Can you work these out from the model? Positions are in its coordinate system, mm. A direction names the side the tool comes from. Give positions to 0.01 mm unless a question says otherwise; leave off trailing zeros. Write each loop counter-clockwise with the first axis right and the second up, starting at its lowest first coordinate (ties: lowest second). Pieces come first, ordered by that corner, then holes.
Autodesk Inventor part; units mm, degrees
ref_plane "YZ Plane" through (0, 0, 0) normal (1, 0, 0) x (0, 1, 0)
ref_plane "XZ Plane" through (0, 0, 0) normal (0, 1, 0) x (-1, 0, 0)
ref_plane "XY Plane" through (0, 0, 0) normal (0, 0, 1) x (1, 0, 0)
sketch "Sketch1" plane through (0, 0, 0) normal (1, 0, 0) x (0, 1, 0)
  line L0 (-39.3892, -105) -> (-110, -20.8494)
  line L1 (-110, -20.8494) -> (-110, 0)
  line L2 (-110, 0) -> (0, 0)
  line L3 (0, 0) -> (0, -105)
  line L4 (0, -105) -> (-39.3892, -105)
  line L5 (-110, -20.8494) -> (-119.38, 0) construction
  line L6 (-119.38, 0) -> (-110, 0) construction
  line L7 (-50.8, -25.4) -> (0, -25.4) construction
  line L8 (0, -25.4) -> (0, 0) construction
  line L9 (0, 0) -> (-50.8, 0) construction
  line L10 (-50.8, 0) -> (-50.8, -25.4) construction
  line L11 (-50.8, -25.4) -> (0, 0) construction
  line L12 (0, -25.4) -> (-50.8, 0) construction
  circle A0 centre (-12.7, -12.7) radius 3
  circle A1 centre (-38.1, -12.7) radius 3
  circle A2 centre (-25.4, -75) radius 14.2875
  circle A3 centre (-25.4, -75) radius 30
  line L13 (-50.8, -90.9637) -> (-50.8, -59.0363)
  line L14 (-50.8, -25.4) -> (0, -25.4)
  line L15 (-66.8394, 0) -> (-50.8, -90.9637)
  line L16 (-50.8, -25.4) -> (-50.8, 0)
  point P0 (-25.4, -12.7)
  point P1 (-25.4, -25.4)
  point P2 (-50.8, -75)
  point P3 (0, -90.9637)
  point P4 (0, -25.4)
  point P5 (-50.8, 0)
  dimension "d0" = 50
  dimension "d1" = 119.38
  dimension "d2" = 50.8
  dimension "d3" = 25.4
  dimension "d4" = 25.4
  dimension "d5" = 12.7
  dimension "d6" = 6
  dimension "d7" = 6
  dimension "d11" = 75
  dimension "d13" = 110
  dimension "d16" = 60
  dimension "d17" = 25.4
  dimension "d18" = 25.4
  dimension "d31" = 28.575
  dimension "d33" = 10
extrude "Plate1" add sketch "Sketch1" along normal blind 1.5875 contours A3 L13 L3 | L15 A3 L13 | L15 L2 L16 L14 L3 A3
fillet "Corner Round2" radius 6 4 edges at (0.7937, 0, -90.9637) (0.7937, -50.8, -90.9637) (0.7937, 0, -25.4) (0.7937, -66.8394, 0)
sketch "Sketch3" plane through (0, -50.8, -26.9875) normal (0, 0, 1) x (1, 0, 0)
  line L0 (0, 44.8) -> (0, 1.5875)
  line L1 (0, 1.5875) -> (20, 1.5875)
  line L2 (20, 1.5875) -> (20, 44.8)
  line L3 (20, 44.8) -> (0, 44.8)
edge flange "Flange1" height 20 angle 90 thickness 1.5875 bend radius 1.5875 thickness toward (0, 0, 1) relief straight relief width 1.5875 relief depth 0.7937 edges at (1.5875, -28.4, -25.4) wall of the first edge with corners at (0, -6, -26.9875) (0, -49.2125, -26.9875) (20, -49.2125, -26.9875) (20, -6, -26.9875)
bend "Bend1"
corner "Corner1"
sketch "Sketch4" plane through (1.5875, 0, 0) normal (1, 0, 0) x (0, 0, -1)
  circle A0 centre (75, -25.4) radius 14.2875
  point P0 (0, 0)
  point P1 (100.4, -25.4)
  point P2 (92.9605, -7.4395)
  point P3 (75, 0)
  point P4 (57.0395, -7.4395)
  point P5 (49.6, -25.4)
  point P6 (57.0395, -43.3605)
  point P7 (75, -50.8)
  point P8 (92.9605, -43.3605)
  dimension "d45" = 25.4
  dimension "d48" = 360
hole "Hole2" at (1.5875, -25.4, -100.4) at (1.5875, -7.4395, -92.9605) at (1.5875, -7.4395, -57.0395) at (1.5875, -25.4, -49.6) at (1.5875, -43.3605, -57.0395) at (1.5875, -43.3605, -92.9605) direction (-1, 0, 0) diameter 5.105 depth 1.5875 tip angle 118
sketch "Sketch5" plane through (20, -49.2125, -26.9875) normal (0, 0, -1) x (-1, 0, 0)
  line L0 (0, 0) -> (16.825, 0)
  line L1 (16.825, 0) -> (16.825, 43.2125)
  point P0 (20, 49.2125)
  point P1 (8.9807, 9.8425)
  point P2 (8.9807, 35.2425)
  point P3 (8.4125, 0)
  point P4 (8.9807, 23.8125)
  dimension "d57" = 25.4
  dimension "d58" = 9.8425
  dimension "d67" = 23.8125
  dimension "d68" = 7.8443
hole "Hole3" at (11.0193, -39.37, -26.9875) at (11.0193, -13.97, -26.9875) at (11.0193, -25.4, -26.9875) direction (0, 0, 1) diameter 5.105 end through all
fillet "Corner Round3" radius 6 2 edges at (20, -49.2125, -26.1938) (20, -6, -26.1937)
sketch "Sketch6" plane through (1.5875, 0, 0) normal (1, 0, 0) x (0, 0, -1)
  line L0 (29.3688, -50.8) -> (0, -50.8)
  line L1 (0, -59.6888) -> (0, -50.8)
  point P0 (0, 0)
  point P1 (12.7, -57.15)
  dimension "d69" = 6.35
  dimension "d70" = 12.7
hole "Hole4" at (1.5875, -57.15, -12.7) direction (-1, 0, 0) diameter 5.105 end through all
equation "\"d7\" = d6"
equation "\"d55\" = Thickness"
equation "\"d76\" = Thickness"
equation "\"d14\" = Thickness"
equation "\"d35\" = BendReliefWidth"
equation "\"d36\" = BendReliefDepth"
equation "\"d37\" = MinimumRemnant"
equation "\"d38\" = TransitionRadius"
equation "\"d41\" = BendRadius"
equation "\"d42\" = CornerReliefSize"
equation "\"d43\" = GapSize"
equation "\"d44\" = JacobiRadiusSize"
equation "\"BendRadius\" = Thickness"
equation "\"BendReliefWidth\" = Thickness"
equation "\"BendReliefDepth\" = 0.5 * Thickness"
equation "\"CornerReliefSize\" = 4 * Thickness"
equation "\"MinimumRemnant\" = 2 * Thickness"
equation "\"TransitionRadius\" = BendRadius"
equation "\"JacobiRadiusSize\" = BendRadius"
equation "\"GapSize\" = Thickness"
properties part number "INSIDE_INTAKE_PLATE_MOTOR_MOUNT" material "Aluminum, 6061-T6"
(1) If I drill on L1, parallel to X at y = -54.5, z = -55.5; L2, parallel to Z at x = 14.25, y = -14; L3, parallel to Y at x = 1.5, z = -74, over which ranges is the centre line in solid material (lowest first)?
Returned:
L1: x = 0 to 1.59
L2: z = -26.99 to -25.4
L3: y = -53.79 to -39.65, -11.15 to 0
(2) If we mould it in two halves opening along Y, with no side actions, what happens to faces 1 (the face through (0.8, -25.3, -105)), 2 (the face through (0.783, -54.658, -12.147)), 3 (the face through (10.91, -16.52, -26.18)), 4 (the face through (0.78, -58.41, -47.81))? For each: +Y half, -Y half, draft (parallel to the pull), parting line (faces both ways), or undercut.
Returned:
face 1: parting line
face 2: undercut
face 3: undercut
face 4: -Y half
(3) For faces 5 (the face through (18.289, -7.804, -26.183)), 6 (the face through (7, -6, -26)), 7 (the face through (0.95, -27.91, -26.31)), which set-ups out of +Z, -Z, +X, -X, +Y, -Y let a thin tool reach every point of the face, with its end or its side?
Returned:
face 5: +Z, -Z, +X, +Y
face 6: +Z, +X, -X
face 7: +Z, -X
(4) Imagine slicing it at B-B, the plane z = -12.7. Write out the boundary of the cut face in (x, y).
Returned:
outline: (0, -64.6) - (1.59, -64.6) - (1.59, -59.7) - (0, -59.7) - close; (0, -54.6) - (1.59, -54.6) - (1.59, -50.8) - (0, -50.8) - close
(5) Imagine slicing it at C-C, the plane y = -57.15. Write out the boundary of the cut face in (x, z).
Returned:
outline: (0, -54.95) - (1.59, -54.95) - (1.59, -15.25) - (0, -15.25) - close; (0, -10.15) - (1.59, -10.15) - (1.59, 0) - (0, 0) - close
(6) Will these pins go through, and if not, where does the flat tip stop? P1, Ø5, axis at x = 4, z = -21.5, coming from the -Y side; P2, Ø6, axis at x = 4, z = -16, coming from the -Y side; P3, Ø8, axis at y = -25.4, z = -49.6, coming from the +X side.
Returned:
P1: stops at y = -63.16
P2: stops at y = -64.33
P3: stops at x = 1.59
(7) Imagine slicing it at D-D, the plane x = 16. Write out the boundary of the cut face in (y, z), plus the area to 3 significant figures.
Returned:
outline: (-48.87, -26.99) - (-6.34, -26.99) - (-6.34, -25.4) - (-48.87, -25.4) - close
area: 67.5 mm2
(8) Imagine slicing it at A-A, the plane y = -25.4. Give the number of separate pieces and of enclosed holes in the cut face, plus the area to 3 significant figures.
Returned:
separate pieces: 5
enclosed holes: 0
area: 84.3 mm2
